For this review, use the dimensioned drawing (mm, ordinates from the lowest corner) and the shaded views. A direction names the side the tool comes from. Round coordinates to 2 decimals unless told otherwise and drop trailing zeros. Loops run counter-clockwise (first coordinate to the right, second up) from the corner with the lowest first, then second, coordinate; pieces in that order, holes last. Notation, with made-up numbers: (24, 16) -> (69, 16) arc R15 ccw to (69, 36) -> close; hole circle Ø6 at (80.25, 44.25). An arc over 180 degrees is marked (long way). Answer as CSV lines item,"result". Start each with the question number.
(1) Draft analysis for pull direction X (two halves, no side actions). For the marked faces 3, 4, 5 and 6, state which applies: +X half, -X half, draft (parallel to the pull), parting line (faces both ways), or undercut.
(2) To check wall thickness, follow line 1 (Z direction, x = 27, y = 13); line 2 (Y direction, x = 20, z = 5); line 3 (Y direction, x = 18.5, z = 17.5). State the ranges of each line that lie inside material, in increasing order. Write a range as from..to.
(3) Take a section at C-C, the plane x = 32.5. Write out the cut boundary in (y, z), and give its area (3 significant figures).
(4) Machinability: for the marked faces 1 and 2, which of the approach directions +Z, -Z, +X, -X, +Y, -Y give a long, thin tool a straight path to every point of the face, cutting with its end or side? Answer none if there is none.
(5) Take a section at A-A, the plane x = 20. Write out the cut boundary in (y, z), and give its area (3 significant figures).
(6) For P1, Ø3, axis at x = 22.5, y = 28, coming from the +Z side; P2, Ø12.5, axis at x = 10.5, z = 24, coming from the +Y side, all flat-tipped, find the tip position at first contact; note any pin that passes through.
(7) Take a section at D-D, the plane z = 16. Write out the cut boundary in (x, y), and give its area (3 significant figures).
(8) Take a section at B-B, the plane y = 17.5. Write out the cut boundary in (x, z) (1 decimal).
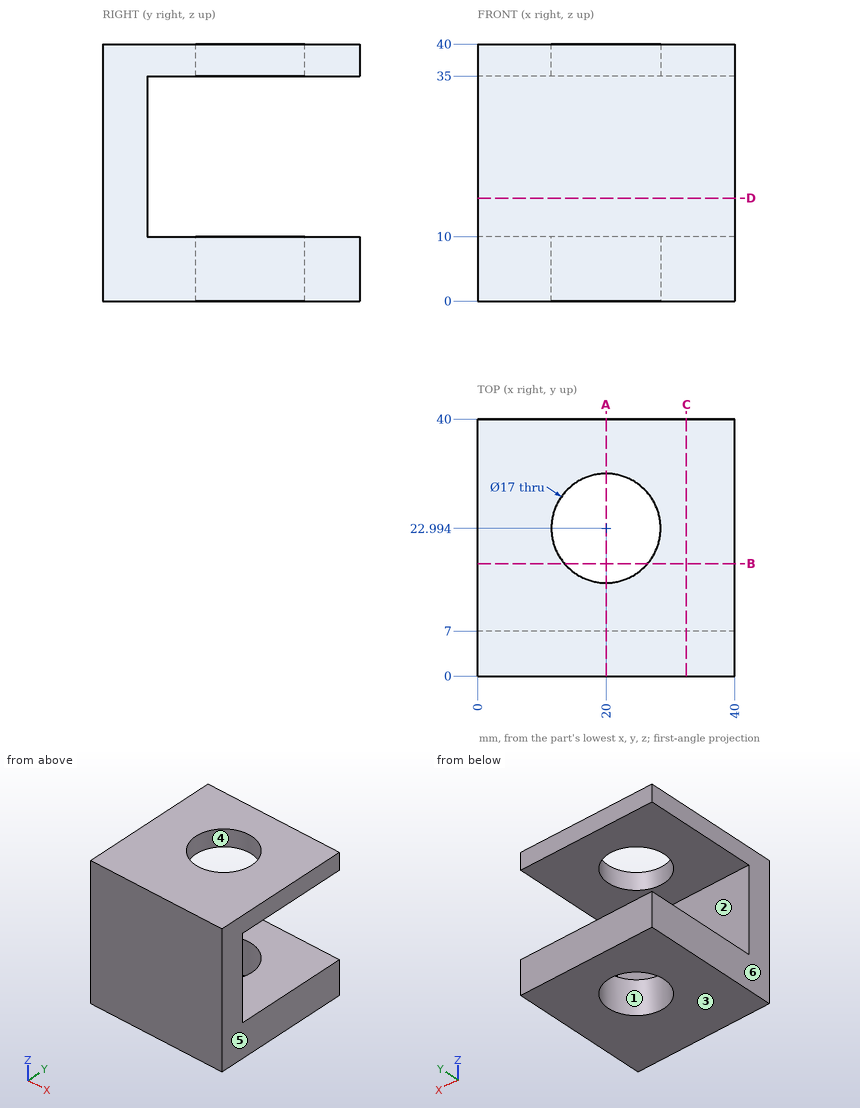
The answers:
1,face 3,"draft"
1,face 4,"undercut"
1,face 5,"+X half"
1,face 6,"-X half"
2,line 1,"0..10, 35..40"
2,line 2,"0..14.49, 31.49..40"
2,line 3,"0..7"
3,outline,"(0, 0) -> (40, 0) -> (40, 10) -> (7, 10) -> (7, 35) -> (40, 35) -> (40, 40) -> (0, 40) -> close"
3,area,"775 mm²"
4,face 1,"+Z, -Z"
4,face 2,"+X, -X, +Y"
5,outline,"(0, 0) -> (14.49, 0) -> (14.49, 10) -> (7, 10) -> (7, 35) -> (14.49, 35) -> (14.49, 40) -> (0, 40) -> close; (31.49, 0) -> (40, 0) -> (40, 10) -> (31.49, 10) -> close; (31.49, 35) -> (40, 35) -> (40, 40) -> (31.49, 40) -> close"
5,area,"520 mm²"
6,P1,"through"
6,P2,"y = 7"
7,outline,"(0, 0) -> (40, 0) -> (40, 7) -> (0, 7) -> close"
7,area,"280 mm²"
8,outline,"(0, 0) -> (13.5, 0) -> (13.5, 10) -> (0, 10) -> close; (0, 35) -> (13.5, 35) -> (13.5, 40) -> (0, 40) -> close; (26.5, 0) -> (40, 0) -> (40, 10) -> (26.5, 10) -> close; (26.5, 35) -> (40, 35) -> (40, 40) -> (26.5, 40) -> close"
